Input: dimensioned drawing with shaded views. Units: mm. Origin: part minimum x, y, z. Round coordinates to 2 decimals unless told otherwise and drop trailing zeros. Loops run counter-clockwise (first coordinate to the right, second up) from the corner with the lowest first, then second, coordinate; pieces in that order, holes last.
Item 1: Section query A-A on z = 50. Return loops of the section in (x, y).
Item 2: Ray query, L1, parallel to Z at x = 112.2, y = 10.25; L2, parallel to Z at x = 285, y = 5; L3, parallel to Z at x = 16, y = 16. Return the intervals inside material, ascending.
Item 3: First-contact query: P1, Ø17.5, axis at x = 15, z = 85, coming from the +Y side; P2, Ø5.5, axis at x = 112.2, z = 87.8, coming from the -Y side. Flat tips, straight axial feed; report the tip coordinate or a pass-through.
Item 4: Section query B-B on x = 285. Return loops of the section in (y, z).
Item 5: Section query C-C on y = 10. Give the number of separate pieces and of enclosed holes in the cut face, then the cut area to 3 significant figures.
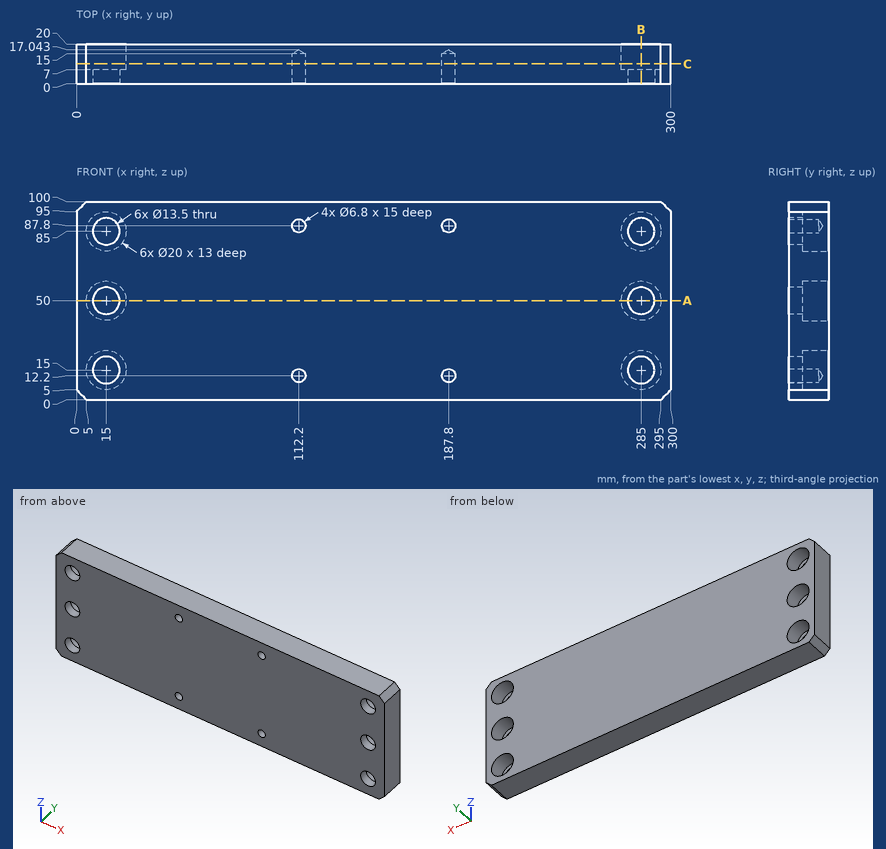
Data:
1. outline: (0, 0) - (8.25, 0) - (8.25, 7) - (5, 7) - (5, 20) - (0, 20) - close; (21.75, 0) - (278.25, 0) - (278.25, 7) - (275, 7) - (275, 20) - (25, 20) - (25, 7) - (21.75, 7) - close; (291.75, 0) - (300, 0) - (300, 20) - (295, 20) - (295, 7) - (291.75, 7) - close
2. L1: z = 0 to 8.8, 15.6 to 84.4, 91.2 to 100
2. L2: z = 0 to 8.25, 21.75 to 43.25, 56.75 to 78.25, 91.75 to 100
2. L3: z = 0 to 5.05, 24.95 to 40.05, 59.95 to 75.05, 94.95 to 100
3. P1: stops at y = 7
3. P2: stops at y = 15.39
4. outline: (0, 0) - (20, 0) - (20, 5) - (7, 5) - (7, 8.25) - (0, 8.25) - close; (0, 21.75) - (7, 21.75) - (7, 25) - (20, 25) - (20, 40) - (7, 40) - (7, 43.25) - (0, 43.25) - close; (0, 56.75) - (7, 56.75) - (7, 60) - (20, 60) - (20, 75) - (7, 75) - (7, 78.25) - (0, 78.25) - close; (0, 91.75) - (7, 91.75) - (7, 95) - (20, 95) - (20, 100) - (0, 100) - close
5. separate pieces: 1
5. enclosed holes: 10
5. area: 27,900 mm2
